Geometry check sheet. Reference: the model listing, model coordinates, mm. A direction names the side the tool comes from. Give positions to 0.01 mm unless a question says otherwise; leave off trailing zeros. Order: outer loops, then holes, each group sorted by start corner. A loop starts at its lowest first (then second) coordinate and runs counter-clockwise, first axis right, second up. Notation, with made-up numbers: M 28.5,61.5 L 46.5,61.5 A33 ccw 46.5,99.5 Z; hole C -31,-9.5 d8. An arc over 180 degrees is marked long. Answer as CSV lines item,"result". Start each with the question number.
Q1. Section check D-D, the plane y = 2.25. Record the boundary of the cut face in (x, z).
Q2. Section check B-B, the plane y = 0. Record the boundary of the cut face in (x, z).
Q3. Set-up check for faces 1 (the flat face through (-17.8, 0, -9)), 2 (the flat face through (-16.212, 0, -8)): record each of +Z, -Z, +X, -X, +Y, -Y from which the full face is reachable in a straight line by a thin tool's end or side.
Q4. Go/stop test with flat-tipped pins: pin 1 (1.5 mm diameter, centred on y = -1, z = -14.5, fed in from +X); pin 2 (3 mm diameter, centred on x = 1.5, z = -14, fed in from +Y); pin 3 (3 mm diameter, centred on x = -4.5, y = -1.5, fed in from +Z). Record where each tip stops, or that it passes through.
Q5. Thickness scan on line 1 (Y direction, x = -17.2, z = 0); line 2 (X direction, y = 1.5, z = -8). Record the ranges inside material, lowest first.
Q6. Section check C-C, the plane x = 0. Record the boundary of the cut face in (y, z).
Q7. Mould release check, pull along Y, two halves, no side actions. Record for faces 3 (the flat face through (-8, 0, -16.212)), 4 (the flat face through (-17, 3.75, -12)), 5 (the cylindrical face through (-3, 0, -17)), 6 (the cylindrical face through (-17, 0, 3)): +Y half, -Y half, draft (parallel to the pull), parting line (faces both ways), or undercut.
Q8. Section check A-A, the plane z = 0. Record the boundary of the cut face in (x, y).
```python
from build123d import *

# Parameters (mm, degrees)
BOSS_EXTRUDE1_DEPTH = 3.75
SKETCH2_R           = 3
CUT_EXTRUDE1_DEPTH  = 28.192786842
SKETCH3_R           = 3
CUT_EXTRUDE2_DEPTH  = 28.192786842


with BuildPart() as part:
    # Sketch1 → Boss-Extrude1 (new, symmetric)
    with BuildSketch(Plane(origin=(0, 0, 0), x_dir=(1, 0, 0), z_dir=(0, 1, 0))):
        Polygon((-4, 16.2125), (4, 16.2125), (4, 17.8), (-4, 17.8), (-17.8, 17.8), (-17.8, 4), (-17.8, -4), (-16.2125, -4), (-16.2125, 4), (-16.2125, 16.2125), align=None)
    extrude(amount=BOSS_EXTRUDE1_DEPTH, both=True)

    # Sketch2 → Cut-Extrude1 (cut, through all)
    with BuildSketch(Plane.XY.offset(-16.2125)):
        Circle(SKETCH2_R)
    extrude(amount=-CUT_EXTRUDE1_DEPTH, mode=Mode.SUBTRACT)

    # Sketch3 → Cut-Extrude2 (cut, through all)
    with BuildSketch(Plane(origin=(-16.2125, 0, 0), x_dir=(0, 0, -1), z_dir=(1, 0, 0))):
        Circle(SKETCH3_R)
    extrude(amount=-CUT_EXTRUDE2_DEPTH, mode=Mode.SUBTRACT)


solid = part.part
```
Answer block:
1,outline,"M -17.8,-17.8 L -1.98,-17.8 L -1.98,-16.21 L -16.21,-16.21 L -16.21,-1.98 L -17.8,-1.98 Z; M -17.8,1.98 L -16.21,1.98 L -16.21,4 L -17.8,4 Z; M 1.98,-17.8 L 4,-17.8 L 4,-16.21 L 1.98,-16.21 Z"
2,outline,"M -17.8,-17.8 L -3,-17.8 L -3,-16.21 L -16.21,-16.21 L -16.21,-3 L -17.8,-3 Z; M -17.8,3 L -16.21,3 L -16.21,4 L -17.8,4 Z; M 3,-17.8 L 4,-17.8 L 4,-16.21 L 3,-16.21 Z"
3,face 1,"+Z, -Z, -X, +Y, -Y"
3,face 2,"+Z, +X, +Y, -Y"
4,pin 1,"stops at x = -16.21"
4,pin 2,"passes through"
4,pin 3,"stops at z = -16.21"
5,line 1,"y = -3.75 to -3, 3 to 3.75"
5,line 2,"x = -17.8 to -16.21"
6,outline,"M -3.75,-17.8 L -3,-17.8 L -3,-16.21 L -3.75,-16.21 Z; M 3,-17.8 L 3.75,-17.8 L 3.75,-16.21 L 3,-16.21 Z"
7,face 3,"draft"
7,face 4,"+Y half"
7,face 5,"undercut"
7,face 6,"undercut"
8,outline,"M -17.8,-3.75 L -16.21,-3.75 L -16.21,-3 L -17.8,-3 Z; M -17.8,3 L -16.21,3 L -16.21,3.75 L -17.8,3.75 Z"
